Work out the finished part from the listing and answer in its coordinate system (mm). A direction names the side the tool comes from. Coordinates: 2 decimals unless noted, no trailing zeros. Loops run counter-clockwise (first coordinate to the right, second up) from the corner with the lowest first, then second, coordinate; pieces in that order, holes last. Notation, with made-up numbers: (63, 70) - (96, 70) arc R23 cw to (96, 106) - close; hole circle Ø2 at (64, -31). An arc over 180 degrees is marked (long way). Write each question's results on one line, items separated by ' | '. Start each with the question number.
1. A cutting plane is placed at D-D on x = 7. Determine the outline of the cut face in (y, z) (3 decimals), then the cut area to 3 significant figures.
2. Find the intervals of material crossed by line 1 along Z through (x, y) = (26, 7.25); line 2 along Z through (x, y) = (20, 2); line 3 along X through (y, z) = (7.25, -21), in increasing order. Write a range as [from, to].
3. A cutting plane is placed at B-B on z = -12. Determine the outline of the cut face in (x, y) (3 decimals), then the cut area to 3 significant figures.
4. A cutting plane is placed at C-C on y = -1. Determine the outline of the cut face in (x, z).
5. Each of these flat-tipped pins is pushed along its axis until it touches: P1, Ø5, axis at y = 7.14, z = 42.07, coming from the +X side; P2, Ø3, axis at x = 17, y = 0, coming from the +Z side; P3, Ø15.5, axis at x = -9.5, z = 4, coming from the +Y side; P4, Ø1, axis at x = 17.5, y = 6.5, coming from the +Z side. Where does it stop, or does it pass through?
6. Determine the mould class of faces 5 (the flat face through (0, -3.175, 1)), 6 (the flat face through (0, 5, 38.894)), 7 (the flat face through (0, 0, 42.069)) for opening direction Z: released by +Z, released by -Z, zero draft, split by the parting line, or undercut.
7. Which of the six approach directions +Z, -Z, +X, -X, +Y, -Y give full straight-line access (tool end or side, diameter ignored) to faces 1 (the flat face through (-0.41, 10.23, 40.37)), 2 (the cylindrical face through (20.914, 6.178, 40.809)), 3 (the flat face through (0, 5, -38.894)), 4 (the cylindrical face through (-0.18, 8.19, 39.07))?
Autodesk Inventor part; units mm, degrees
ref_plane "YZ Plane" through (0, 0, 0) normal (1, 0, 0) x (0, 1, 0)
ref_plane "XZ Plane" through (0, 0, 0) normal (0, 1, 0) x (-1, 0, 0)
ref_plane "XY Plane" through (0, 0, 0) normal (0, 0, 1) x (1, 0, 0)
sketch "Sketch2" plane through (0, 0, 0) normal (0, 1, 0) x (-1, 0, 0)
  line L0 (29.3687, 42.0688) -> (-29.3688, 42.0688)
  line L1 (-29.3688, 42.0688) -> (-29.3687, -42.0688)
  line L2 (-29.3687, -42.0688) -> (29.3688, -42.0688)
  line L3 (29.3688, -42.0688) -> (29.3687, 42.0688)
  line L4 (29.3687, 42.0688) -> (-29.3687, -42.0688) construction
  line L5 (-29.3688, 42.0688) -> (29.3688, -42.0688) construction
  point P0 (0, 0)
  dimension "d4" = 58.7375
  dimension "d5" = 84.1375
extrude "Extrusion1" add sketch "Sketch2" against normal blind 3.175
sketch "Sketch3" plane through (0, 0, 0) normal (0, 1, 0) x (1, 0, 0)
  line L0 (29.3688, -42.0688) -> (-29.3687, -42.0688)
  line L1 (-29.3688, 42.0688) -> (29.3687, 42.0688)
  line L2 (-29.3687, -42.0688) -> (29.3687, -42.0688)
  line L3 (29.3687, -42.0688) -> (29.3687, 42.0688)
  line L4 (29.3687, 42.0688) -> (-29.3687, 42.0688)
  line L5 (-29.3687, 42.0688) -> (-29.3687, -42.0688)
  line L6 (-26.1938, -38.8937) -> (26.1937, -38.8937)
  line L7 (26.1937, -38.8937) -> (26.1937, 38.8937)
  line L8 (26.1937, 38.8937) -> (-26.1938, 38.8937)
  line L9 (-26.1938, 38.8937) -> (-26.1938, -38.8937)
  line L10 (-26.1938, -38.8937) -> (26.1937, 38.8937) construction
  line L11 (26.1937, -38.8937) -> (-26.1938, 38.8937) construction
  point P0 (0, 0)
  dimension "d8" = 3.175
  dimension "d9" = 3.175
extrude "Extrusion2" add sketch "Sketch3" along normal blind 7.1437
sketch "Sketch6" plane through (-29.3688, -3.175, -42.0688) normal (-1, 0, 0) x (0, 0, 1)
  line L0 (0, 10.3187) -> (84.1375, 10.3187)
  line L1 (84.1375, 10.3187) -> (84.1375, 0)
  circle A0 centre (84.1375, 10.3187) radius 3.175
  point P0 (42.0688, 3.175)
  dimension "d16" = 6.35
extrude "Extrusion5" add sketch "Sketch6" against normal blind 58.7375
sketch "Sketch8" plane through (-29.3688, -3.175, -42.0688) normal (-1, 0, 0) x (0, 0, 1)
  arc A0 (84.1375, 7.1437) -> (80.9625, 10.3187) centre (84.1375, 10.3187) ccw
  circle A1 centre (84.1375, 10.3187) radius 1.5875
  point P0 (42.0688, 3.175)
  dimension "d21" = 3.175
extrude "Extrusion6" cut sketch "Sketch8" against normal blind 58.7375
sketch "Sketch11" plane through (0, 7.1437, 0) normal (0, 1, 0) x (1, 0, 0)
  line L0 (-29.3688, 42.0688) -> (29.3687, 42.0688)
  line L1 (-29.3688, 42.0688) -> (29.3687, 42.0688)
  line L2 (29.3687, 42.0688) -> (29.3688, -38.7648)
  line L3 (29.3687, 42.0688) -> (29.3688, -42.0688)
  line L4 (26.1937, -38.8937) -> (29.3688, -38.8937)
  line L5 (26.1937, 38.8937) -> (26.1937, -38.8937)
  line L6 (26.1937, -38.8937) -> (26.1937, 38.8937)
  line L7 (26.1937, 38.8937) -> (-26.1938, 38.8937)
  line L8 (-29.3687, -38.8938) -> (-26.1938, -38.8937)
  line L9 (-26.1938, 38.8937) -> (-26.1938, -38.8937)
  line L10 (-26.1938, -38.8937) -> (-29.3687, -38.8938)
  line L11 (-29.3688, 42.0688) -> (-29.3687, -38.8938)
  line L12 (-29.3687, -38.8938) -> (-29.3688, 42.0688)
  point P0 (0, 0)
extrude "Extrusion9" add sketch "Sketch11" along normal blind 3.175
sketch "Sketch12" plane through (-29.3688, -3.175, -42.0688) normal (-1, 0, 0) x (0, 0, 1)
  line L0 (80.9625, 3.175) -> (80.9625, 10.3187)
  line L1 (80.9625, 10.3187) -> (80.9625, 13.3208)
  arc A0 (84.1375, 7.1437) -> (80.9625, 10.3187) centre (84.1375, 10.3187) ccw
  line L2 (80.9625, 13.3208) -> (83.9598, 13.4888)
  point P0 (42.0688, 3.175)
extrude "Extrusion10" add sketch "Sketch12" against normal blind 58.7375
ref_plane "Work Plane1" through (-0.0063, -3.175, 42.0688) normal (1, 0, 0) x (0, 0, -1)
sketch "Sketch13" plane through (-0.0063, -3.175, 42.0688) normal (1, 0, 0) x (0, 0, -1)
  circle A0 centre (0, 10.3187) radius 1.5875
  circle A1 centre (0, 10.3187) radius 3.175
  point P0 (42.0688, 3.175)
  dimension "d33" = 6.35
extrude "Extrusion11" cut sketch "Sketch13" along normal mid plane 25.4
equation "\"d4\" = 2 * materialWallThickness + cardDeckWidth + cardDeckAirGap"
equation "\"d5\" = 2 * materialWallThickness + cardDeckLength + cardDeckAirGap"
equation "\"d6\" = baseWallThickness"
equation "\"d8\" = baseWallThickness"
equation "\"d9\" = baseWallThickness"
equation "\"d10\" = 0.5 * cardDeckDepth"
equation "\"d19\" = d4"
equation "\"d22\" = d4"
equation "\"d30\" = d4"
equation "\"cardDeckWidth\" = 50.8"
equation "\"cardDeckLength\" = 76.2"
equation "\"d0\" = cardDeckWidth"
equation "\"d1\" = cardDeckLength"
equation "\"cardDeckDepth\" = 14.2875"
equation "\"d2\" = cardDeckDepth"
equation "\"d3\" = 0"
equation "\"materialWallThickness\" = 3.175"
equation "\"baseWallThickness\" = 3.175"
equation "\"cardDeckAirGap\" = 1.5875"
equation "\"hingeOuterDiam\" = 12.7"
equation "\"hingeInnerDiam\" = 6.35"
properties part number "TopHalfOfBoard" material "ABS Plastic"
Values:
1) outline: (-3.175, -42.069) - (10.319, -42.069) - (10.319, -38.894) - (0, -38.894) - (0, 38.894) - (10.146, 38.894) - (10.314, 41.891) arc R3.175 cw to (3.969, 42.069) - (-3.175, 42.069) - close | area: 317 mm^2
2) line 1: [-42.07, -38.89], [38.89, 40.48], [43.65, 45.24] | line 2: [-42.07, -38.89], [38.89, 42.07] | line 3: [-29.37, -26.19], [26.19, 29.37]
3) outline: (-29.369, -3.175) - (29.369, -3.175) - (29.369, 10.319) - (26.194, 10.319) - (26.194, 0) - (-26.194, 0) - (-26.194, 10.319) - (-29.369, 10.319) - close | area: 252 mm^2
4) outline: (-29.37, -42.07) - (29.37, -42.07) - (29.37, 42.07) - (-29.37, 42.07) - close
5) P1: x = 29.37 | P2: z = 42.07 | P3: y = 0 | P4: z = 45.24
6) face 5: zero draft | face 6: undercut | face 7: released by +Z
7) face 1: +X, -X, +Y | face 2: +X, -X | face 3: +Y | face 4: +Z
